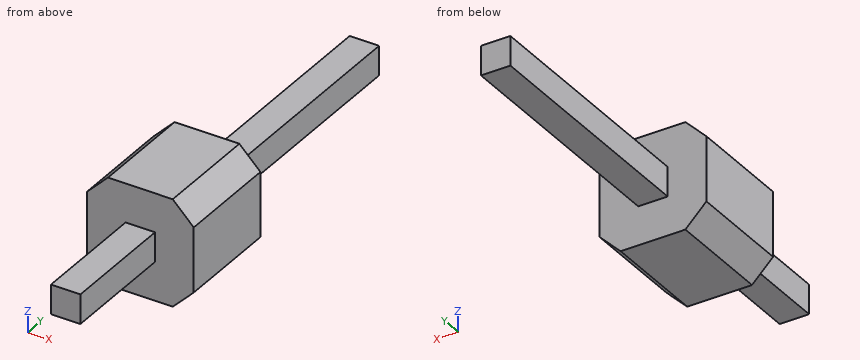
```python
from build123d import *

# Parameters (mm, degrees)
SKETCH1_W           = 0.7
SKETCH1_H           = 0.7
BOSS_EXTRUDE1_DEPTH = 11.2
BOSS_EXTRUDE2_START = 2.8
SKETCH1_3_W         = 2.54
SKETCH1_3_H         = 2.54
SKETCH1_3_W_2       = 0.7
SKETCH1_3_H_2       = 0.7
BOSS_EXTRUDE2_DEPTH = 2.5
CHAMFER1_SIZE       = 0.5


with BuildPart() as part:
    # Sketch1 → Boss-Extrude1 (new body)
    with BuildSketch(Plane(origin=(0, 0, 0), x_dir=(1, 0, 0), z_dir=(0, 1, 0))):
        with Locations((1.27, 1.27)):
            Rectangle(SKETCH1_W, SKETCH1_H)
    extrude(amount=BOSS_EXTRUDE1_DEPTH)

    # Sketch1<3> → Boss-Extrude2 (add)
    with BuildSketch(Plane(origin=(0, 0, 0), x_dir=(1, 0, 0), z_dir=(0, 1, 0)).offset(BOSS_EXTRUDE2_START)):
        with Locations((1.27, 1.27)):
            Rectangle(SKETCH1_3_W, SKETCH1_3_H)
        with Locations((1.27, 1.27)):
            Rectangle(SKETCH1_3_W_2, SKETCH1_3_H_2, mode=Mode.SUBTRACT)
    extrude(amount=BOSS_EXTRUDE2_DEPTH)

    # Chamfer1
    chamfer1_edges = [part.edges().sort_by_distance(p)[0] for p in [
        (0, 4.05, 0),
        (2.54, 4.05, 0),
        (2.54, 4.05, -2.54),
        (0, 4.05, -2.54),
    ]]
    chamfer(chamfer1_edges, length=CHAMFER1_SIZE)


solid = part.part
```
Can you work these out from the model? Positions are in its coordinate system, mm. Coordinates: 2 decimals unless noted, no trailing zeros. Loops run counter-clockwise (first coordinate to the right, second up) from the corner with the lowest first, then second, coordinate; pieces in that order, holes last. Notation, with made-up numbers: (10, -8.75) - (59, -8.75) arc R17 ccw to (59, 4.25) - close; hole circle Ø6 at (85, 17). An arc over 180 degrees is marked (long way). Use a Markdown table: item, result.
Item 1: I want a section at B-B on x = 1.3. Please give me the cut outline in (y, z).
Numbers:
| item | result |
|---|---|
| outline | (0, -1.62) - (2.8, -1.62) - (2.8, -2.54) - (5.3, -2.54) - (5.3, -1.62) - (11.2, -1.62) - (11.2, -0.92) - (5.3, -0.92) - (5.3, 0) - (2.8, 0) - (2.8, -0.92) - (0, -0.92) - close |
Item 2: If I drill on probe 1 along Z at (x, y) = (1.5, 2.25); probe 2 along X at (y, z) = (9.25, -1.3); probe 3 along Y at (x, z) = (1, -0.6), over which ranges is the centre line in solid material (lowest first)? Write a range as from..to.
Numbers:
| item | result |
|---|---|
| probe 1 | z = -1.62..-0.92 |
| probe 2 | x = 0.92..1.62 |
| probe 3 | y = 2.8..5.3 |
Item 3: I want a section at D-D on x = 0.7. Please give me the cut outline in (y, z), and give its area (3 significant figures).
Numbers:
| item | result |
|---|---|
| outline | (2.8, -2.54) - (5.3, -2.54) - (5.3, 0) - (2.8, 0) - close |
| area | 6.35 mm2 |
Item 4: I want a section at C-C on y = 3.5. Please give me the cut outline in (x, z), and give its area (3 significant figures).
Numbers:
| item | result |
|---|---|
| outline | (0, -2.04) - (0.5, -2.54) - (2.04, -2.54) - (2.54, -2.04) - (2.54, -0.5) - (2.04, 0) - (0.5, 0) - (0, -0.5) - close |
| area | 5.95 mm2 |
Item 5: Will these pins go through, and if not, where does the flat tip stop? pin 1 (0.8 mm diameter, centred on x = 1.5, y = 7.5, fed in from -Z); pin 2 (0.6 mm diameter, centred on y = 1, z = -1, fed in from -X).
Numbers:
| item | result |
|---|---|
| pin 1 | stops at z = -1.62 |
| pin 2 | stops at x = 0.92 |
Item 6: I want a section at A-A on z = -1.2. Please give me the cut outline in (x, y).
Numbers:
| item | result |
|---|---|
| outline | (0, 2.8) - (0.92, 2.8) - (0.92, 0) - (1.62, 0) - (1.62, 2.8) - (2.54, 2.8) - (2.54, 5.3) - (1.62, 5.3) - (1.62, 11.2) - (0.92, 11.2) - (0.92, 5.3) - (0, 5.3) - close |
